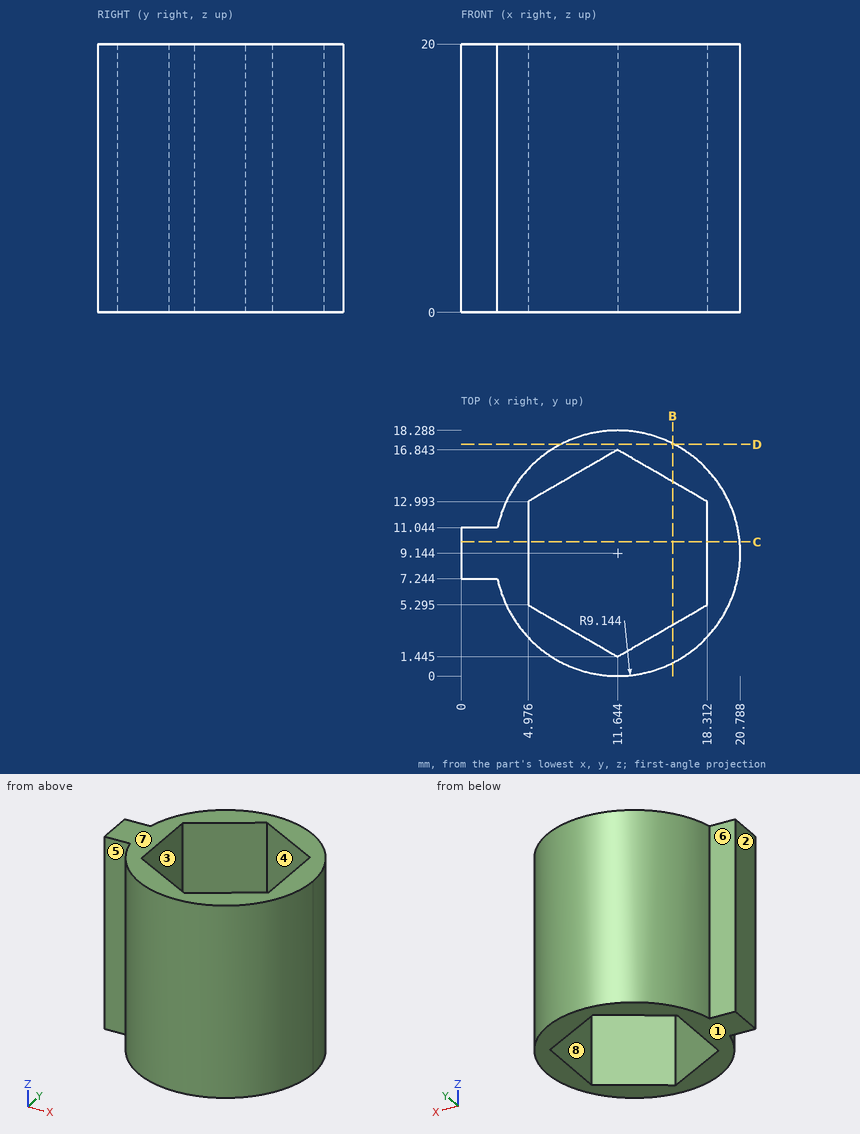
The figure shows three views and two pictorial views of one solid part (mm, origin at its lowest corner). Answer the questions. A direction names the side the tool comes from. Give positions to 0.01 mm unless a question says otherwise; leave off trailing zeros. Write each loop counter-clockwise with the first axis right and the second up, starting at its lowest first coordinate (ties: lowest second). Pieces come first, ordered by that corner, then holes. Notation, with made-up numbers: (36.25, -2) -> (63.25, -2) arc R33 cw to (63.25, 35) -> close; hole circle Ø6 at (75.25, 23.25). An arc over 180 degrees is marked (long way). Write each question's results on one line, items separated by ' | '.
1. Find section D-D on y = 17.25. Determine the outline of the cut face in (x, z) (1 decimal).
Data:
outline: (7.4, 0) -> (15.9, 0) -> (15.9, 20) -> (7.4, 20) -> close
2. Find section C-C on y = 10. Determine the outline of the cut face in (x, z).
Data:
outline: (0, 0) -> (4.98, 0) -> (4.98, 20) -> (0, 20) -> close; (18.31, 0) -> (20.75, 0) -> (20.75, 20) -> (18.31, 20) -> close
3. Each of these flat-tipped pins is pushed along its axis until it touches: pin 1 Ø5 at (y, z) = (10, 3) entering from +X; pin 2 Ø0.8 at (x, z) = (2, 6.5) entering from -Y; pin 3 Ø12 at (x, z) = (3.5, 6.5) entering from +Y; pin 4 Ø3 at (x, z) = (5, 17) entering from +Y (1 decimal). Where does it stop, or does it pass through?
Data:
pin 1: x = 20.79 | pin 2: y = 7.24 | pin 3: y = 18.03 | pin 4: y = 16.7
4. A tool of negligible diameter and unlimited length cuts with its end or side. For the marked faces 5, 6, 7 and 8, from which of +Z, -Z, +X, -X, +Y, -Y can it reach the whole face along a straight path? Write none if from no direction.
Data:
face 5: +Z, -Z, -X, -Y | face 6: +Z, -Z, -X, +Y | face 7: +Z, +X, -X, +Y, -Y | face 8: +Z, -Z
5. Find section B-B on x = 15.75. Determine the outline of the cut face in (y, z) (1 decimal), and give its area (3 significant figures).
Data:
outline: (1, 0) -> (3.8, 0) -> (3.8, 20) -> (1, 20) -> close; (14.5, 0) -> (17.3, 0) -> (17.3, 20) -> (14.5, 20) -> close | area: 114 mm^2
6. Determine the mould class of the marked faces 1, 2, 3 and 4 for opening direction X: +X half, -X half, draft (parallel to the pull), parting line (faces both ways), or undercut.
Data:
face 1: draft | face 2: -X half | face 3: undercut | face 4: undercut
7. Straight lines are drawn through the part: L1, parallel to Y at x = 16, z = 14.5 (1 decimal); L2, parallel to Y at x = 9, z = 4.75 (1 decimal); L3, parallel to X at y = 15.5, z = 6.75 (1 decimal). For each, find the intervals that lie inside material, in ascending order.
Data:
L1: 1.1 to 4, 14.3 to 17.2 | L2: 0.4 to 3, 15.3 to 17.9 | L3: 5.1 to 9.3, 14 to 18.2
